The listing builds one solid part. Answer for the finished solid, in the listing's coordinates (mm). Face numbers are marked on the shaded views. A direction names the side the tool comes from. Give positions to 0.01 mm unless a question says otherwise; leave off trailing zeros. Loops run counter-clockwise (first coordinate to the right, second up) from the corner with the lowest first, then second, coordinate; pieces in that order, holes last. Notation, with made-up numbers: (-39.75, -22.75) - (4.25, -22.75) arc R30 ccw to (4.25, 1.25) - close; hole circle Ø4 at (-10, -9.75). An arc over 180 degrees is marked (long way). Answer as CSV lines item,"result". Start each with the question number.
1) A cutting plane is placed at A-A (z = 64.4). Determine the outline of the cut face in (x, y), and give its area (3 significant figures).
2) A cutting plane is placed at C-C (x = -43.5). Determine the outline of the cut face in (y, z), and give its area (3 significant figures).
3) Flat-ended cylindrical pins translate along their axes: pin 1 (2 mm diameter, centred on x = -46, y = 16.5, fed in from +Z); pin 2 (8 mm diameter, centred on y = 12.5, z = 57.4, fed in from -X); pin 3 (3 mm diameter, centred on y = 26.5, z = 49, fed in from +X). Find the tip coordinate at first contact, or state that the pin passes through.
4) A cutting plane is placed at B-B (y = 20). Determine the outline of the cut face in (x, z).
5) Find the intervals of material crossed by line 1 along Z through (x, y) = (-27.9, -1.5); line 2 along Y through (x, z) = (-27.35, 21); line 3 along X through (y, z) = (-2, 53), in increasing order.
6) A cutting plane is placed at D-D (z = 49). Determine the outline of the cut face in (x, y), and give its area (3 significant figures).
7) For a pull along X with two mould halves and no side action, classify the marked faces 4, 5 and 6 as pulls with the +X half, pulls with the -X half, needs draft (parallel to the pull), parting line crosses it, or undercut.
8) For the marked faces 1, 2 and 3, determine the directions among +Z, -Z, +X, -X, +Y, -Y from which every point of the face is accessible in a straight line to the end or side of a thin tool.
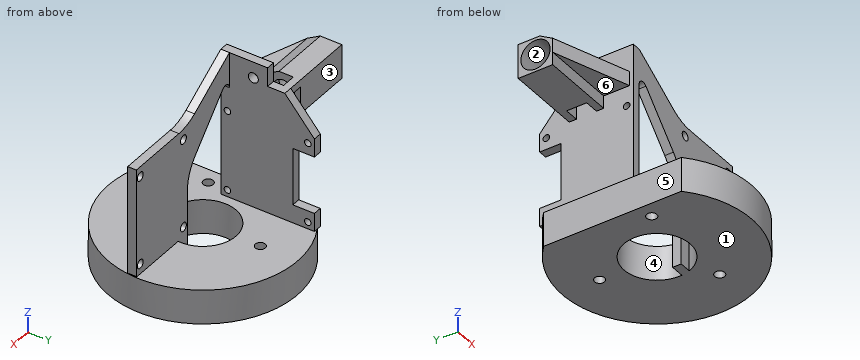
```python
from build123d import *

# Parameters (mm, degrees)
SKETCH_1_R           = 29
EXTRUDE_1_DEPTH      = 5
HOLE_WIZARD_1_D      = 3.5
HOLE_WIZARD_2_D      = 23
EXTRUDE_3_DEPTH      = 65
SKETCH_9_W           = 1
SKETCH_9_H           = 5
CUT_EXTRUDE_1_DEPTH  = 10
SKETCH_10_W          = 3
SKETCH_10_H          = 65
EXTRUDE_5_DEPTH      = 10
HOLE_WIZARD_3_D      = 3.5
EXTRUDE_START        = -65
EXTRUDE_6_DEPTH      = 65
SKETCH_22_W          = 12
SKETCH_22_H          = 6
EXTRUDE_7_DEPTH      = 3
EXTRUDE_8_DEPTH      = 8
HOLE_WIZARD_5_D      = 7
HOLE_WIZARD_5_DEPTH  = 3
SKETCH_27_W          = 5
SKETCH_27_H          = 3.5
CUT_EXTRUDE_3_DEPTH  = 70.598725899
CUT_EXTRUDE_4_REACH  = 94.289
SKETCH_28_W          = 3
SKETCH_28_H          = 3.5
SKETCH_29_R          = 3.5
EXTRUDE_9_DEPTH      = 18
HOLE_WIZARD_6_D      = 10.2
HOLE_WIZARD_6_DEPTH  = 18
SKETCH_32_W          = 26
SKETCH_32_H          = 5
EXTRUDE_10_DEPTH     = 9
CUT_EXTRUDE_5_REACH  = 88.897
SKETCH_36_W          = 32.8
SKETCH_36_H          = 32.6
EXTRUDE_12_DEPTH     = 3
SKETCH_38_R          = 29
CUT_EXTRUDE_7_DEPTH  = 5
SKETCH_39_W          = 17.667068266
SKETCH_39_H          = 15
CUT_EXTRUDE_8_DEPTH  = 13.6
SKETCH_41_R          = 33
EXTRUDE_14_DEPTH     = 12
HOLE_WIZARD_8_D      = 3.5
HOLE_WIZARD_9_D      = 23
HOLE_WIZARD_10_D     = 2.3
SKETCH_53_W          = 20
SKETCH_53_H          = 15
CUT_EXTRUDE_9_DEPTH  = 3
EXTRUDE_16_DEPTH     = 3
SKETCH_56_W          = 3.442096105
SKETCH_56_H          = 51.4
CUT_EXTRUDE_10_DEPTH = 96.777795528
SKETCH_57_W          = 3
SKETCH_57_H          = 1.3
EXTRUDE_17_DEPTH     = 18.6
EXTRUDE_18_DEPTH     = 3
CUT_EXTRUDE_START    = -12
CUT_EXTRUDE_11_DEPTH = 12
SKETCH_63_W          = 26
SKETCH_63_H          = 3
EXTRUDE_21_DEPTH     = 38
HOLE_WIZARD_11_D     = 3
EXTRUDE_22_DEPTH     = 3
CUT_EXTRUDE_START_2  = 4
CUT_EXTRUDE_13_DEPTH = 4
FILLET_1_R           = 15
FILLET_2_R           = 2
EXTRUDE_23_DEPTH     = 12


with BuildPart() as part:
    # 草图1 → 凸台-拉伸1 (new body)
    with BuildSketch(Plane.XY):
        Circle(SKETCH_1_R)
    extrude(amount=EXTRUDE_1_DEPTH)

    # 孔1 (through all)
    with Locations(Plane.XY.offset(5)):
        with Locations((0, 20), (-17.320508076, -10), (17.320508076, -10)):
            Hole(HOLE_WIZARD_1_D / 2)

    # 孔2 (through all)
    with Locations(Plane.XY.offset(5)):
        with Locations((0, 0)):
            Hole(HOLE_WIZARD_2_D / 2)

    # 草图7 → 凸台-拉伸3 (add)
    with BuildSketch(Plane.XY.offset(5)):
        with BuildLine():
            Line((-28.892040426, 2.5), (-28.892040426, -2.5))
            Line((-28.892040426, -2.5), (-11.22497216, -2.5))
            ThreePointArc((-11.22497216, -2.5), (-11.5, 0), (-11.22497216, 2.5))
            Line((-11.22497216, 2.5), (-28.892040426, 2.5))
        make_face()
    extrude(amount=EXTRUDE_3_DEPTH)

    # 草图9 → 切除-拉伸1 (cut)
    with BuildSketch(Plane.XY.offset(5)):
        with Locations((-29.392040426, 0)):
            Rectangle(SKETCH_9_W, SKETCH_9_H)
    extrude(amount=-CUT_EXTRUDE_1_DEPTH, mode=Mode.SUBTRACT)

    # 草图10 → 凸台-拉伸5 (add)
    with BuildSketch(Plane(origin=(0, 2.5, 0), x_dir=(1, 0, 0), z_dir=(0, 1, 0))):
        with Locations((-27.392040426, -37.5)):
            Rectangle(SKETCH_10_W, SKETCH_10_H)
    extrude(amount=EXTRUDE_5_DEPTH)

    # 孔3 (through all)
    with Locations(Plane.ZY.offset(28.892040426)):
        with Locations((10, 7.5), (64.4, 7.5)):
            Hole(HOLE_WIZARD_3_D / 2)

    # 草图20 → 凸台-拉伸6 (add)
    with BuildSketch(Plane.XY.offset(70).offset(EXTRUDE_START)):
        with BuildLine():
            Line((-11.22497216, 2.5), (-11.22497216, -2.5))
            ThreePointArc((-11.22497216, -2.5), (-11.5, 0), (-11.22497216, 2.5))
        make_face()
    extrude(amount=EXTRUDE_6_DEPTH)

    # 草图22 → 凸台-拉伸7 (add)
    with BuildSketch(Plane.ZY.offset(28.892040426)):
        with Locations((57.4, 15.5)):
            Rectangle(SKETCH_22_W, SKETCH_22_H)
    extrude(amount=-EXTRUDE_7_DEPTH)

    # 草图23 → 凸台-拉伸8 (add)
    with BuildSketch(Plane.ZY.offset(28.892040426)):
        Polygon((51.4, 6.5), (60.801923789, 6.5), (63.4, 11), (63.4, 12.5), (63.4, 18.5), (51.4, 18.5), (51.4, 12.5), align=None)
    extrude(amount=EXTRUDE_8_DEPTH)

    # 孔5
    with Locations(Plane.ZY.offset(36.892040426)):
        with Locations((57.4, 12.5)):
            Hole(HOLE_WIZARD_5_D / 2, depth=HOLE_WIZARD_5_DEPTH)

    # 草图27 → 切除-拉伸3 (cut, through all)
    with BuildSketch(Plane(origin=(0, 0, 51.4), x_dir=(-1, 0, 0), z_dir=(0, 0, -1))):
        with Locations((31.392040426, 14.25)):
            Rectangle(SKETCH_27_W, SKETCH_27_H)
        with Locations((31.392040426, 10.75)):
            Rectangle(SKETCH_27_W, SKETCH_27_H)
    extrude(amount=-CUT_EXTRUDE_3_DEPTH, mode=Mode.SUBTRACT)

    # 草图28 → 切除-拉伸4 (cut, up to next)
    with BuildSketch(Plane(origin=(0, 18.5, 0), x_dir=(1, 0, 0), z_dir=(0, 1, 0)), mode=Mode.PRIVATE) as cut_extrude_4_sk1:
        with Locations((-32.392040426, -59.15)):
            Rectangle(SKETCH_28_W, SKETCH_28_H)
    cut_extrude_4_tool1 = extrude(cut_extrude_4_sk1.sketch, amount=-CUT_EXTRUDE_4_REACH, mode=Mode.PRIVATE) & part.part
    # 草图28 → 切除-拉伸4 (cut, up to next)
    with BuildSketch(Plane(origin=(0, 18.5, 0), x_dir=(1, 0, 0), z_dir=(0, 1, 0)), mode=Mode.PRIVATE) as cut_extrude_4_sk2:
        with Locations((-32.392040426, -55.65)):
            Rectangle(SKETCH_28_W, SKETCH_28_H)
    cut_extrude_4_tool2 = extrude(cut_extrude_4_sk2.sketch, amount=-CUT_EXTRUDE_4_REACH, mode=Mode.PRIVATE) & part.part
    add(cut_extrude_4_tool1.solids().sort_by_distance((-32.39204, 18.5, 59.15))[0], mode=Mode.SUBTRACT)
    add(cut_extrude_4_tool2.solids().sort_by_distance((-32.39204, 18.5, 55.65))[0], mode=Mode.SUBTRACT)

    # 草图29 → 凸台-拉伸9 (add)
    # profile 1 of 2: a face of its own
    with BuildSketch(Plane.ZY.offset(36.892040426)):
        Polygon((60.801923789, 6.5), (63.4, 11), (63.4, 18.5), (51.4, 18.5), (51.4, 6.5), align=None)
        with Locations((57.4, 12.5)):
            Circle(SKETCH_29_R, mode=Mode.SUBTRACT)
    # profile 2 of 2: a face of its own
    with BuildSketch(Plane.ZY.offset(36.892040426)):
        with Locations((57.4, 12.5)):
            Circle(SKETCH_29_R)
    extrude(amount=EXTRUDE_9_DEPTH)

    # 孔6
    with Locations(Plane.ZY.offset(54.892040426)):
        with Locations((57.4, 12.5)):
            Hole(HOLE_WIZARD_6_D / 2, depth=HOLE_WIZARD_6_DEPTH)

    # 草图32 → 凸台-拉伸10 (add)
    with BuildSketch(Plane.XZ.offset(-6.5)):
        with Locations((-41.892040426, 58.301923789)):
            Rectangle(SKETCH_32_W, SKETCH_32_H)
    extrude(amount=EXTRUDE_10_DEPTH)

    # 草图33 → 切除-拉伸5 (cut, up to next)
    with BuildSketch(Plane.XY.offset(60.801923789), mode=Mode.PRIVATE) as cut_extrude_5_sk1:
        Polygon((-54.892040426, 6.5), (-28.892040426, -2.5), (-54.892040426, -2.5), align=None)
    cut_extrude_5_tool1 = extrude(cut_extrude_5_sk1.sketch, amount=-CUT_EXTRUDE_5_REACH, mode=Mode.PRIVATE) & part.part
    add(cut_extrude_5_tool1.solids().sort_by_distance((-46.225374, 0.5, 60.801924))[0], mode=Mode.SUBTRACT)

    # 草图36 → 凸台-拉伸12 (add)
    with BuildSketch(Plane.ZY.offset(28.892040426)):
        with Locations((35, 12.5)):
            Rectangle(SKETCH_36_W, SKETCH_36_H)
    extrude(amount=-EXTRUDE_12_DEPTH)

    # 草图38 → 切除-拉伸7 (cut)
    with BuildSketch(Plane(origin=(0, 0, 0), x_dir=(-1, 0, 0), z_dir=(0, 0, -1))):
        Circle(SKETCH_38_R)
    extrude(amount=-CUT_EXTRUDE_7_DEPTH, mode=Mode.SUBTRACT)

    # 草图39 → 切除-拉伸8 (cut)
    with BuildSketch(Plane(origin=(0, 0, 5), x_dir=(-1, 0, 0), z_dir=(0, 0, -1))):
        with Locations((20.058506293, 5)):
            Rectangle(SKETCH_39_W, SKETCH_39_H)
    extrude(amount=-CUT_EXTRUDE_8_DEPTH, mode=Mode.SUBTRACT)

    # 草图41 → 凸台-拉伸14 (add)
    with BuildSketch(Plane(origin=(0, 0, 18.6), x_dir=(-1, 0, 0), z_dir=(0, 0, -1))):
        with Locations(Location((11.22497216, 0, 0), (0, 0, 57.631283974))):
            Circle(SKETCH_41_R)
    extrude(amount=EXTRUDE_14_DEPTH)

    # 孔8 (through all)
    with Locations(Plane(origin=(0, 0, 6.6), x_dir=(-1, 0, 0), z_dir=(0, 0, -1))):
        with Locations((11.22497216, 20), (-6.095535915, -10), (28.545480236, -10)):
            Hole(HOLE_WIZARD_8_D / 2)

    # 孔9 (through all)
    with Locations(Plane(origin=(0, 0, 6.6), x_dir=(-1, 0, 0), z_dir=(0, 0, -1))):
        with Locations((11.22497216, 0)):
            Hole(HOLE_WIZARD_9_D / 2)

    # 孔10 (through all)
    with Locations(Plane.ZY.offset(28.892040426)):
        with Locations((21, 26.5), (49, 26.5), (49, -1.5), (21, -1.5)):
            Hole(HOLE_WIZARD_10_D / 2)

    # 草图53 → 切除-拉伸9 (cut)
    with BuildSketch(Plane.ZY.offset(28.892040426)):
        with Locations((35, 28.8)):
            Rectangle(SKETCH_53_W, SKETCH_53_H)
    extrude(amount=-CUT_EXTRUDE_9_DEPTH, mode=Mode.SUBTRACT)

    # 草图55 → 凸台-拉伸16 (add)
    with BuildSketch(Plane(origin=(-25.892040426, 0, 0), x_dir=(0, 0, -1), z_dir=(1, 0, 0))):
        Polygon((-51.4, 28.8), (-63.4, 18.5), (-51.4, 18.5), align=None)
    extrude(amount=-EXTRUDE_16_DEPTH)

    # 草图56 → 切除-拉伸10 (cut, through all)
    with BuildSketch(Plane(origin=(0, 2.5, 0), x_dir=(1, 0, 0), z_dir=(0, 1, 0))):
        with Locations((-24.170992373, -44.3)):
            Rectangle(SKETCH_56_W, SKETCH_56_H)
    extrude(amount=-CUT_EXTRUDE_10_DEPTH, mode=Mode.SUBTRACT)

    # 草图57 → 凸台-拉伸17 (add)
    with BuildSketch(Plane.XY.offset(51.4)):
        with Locations((-27.392040426, -3.15)):
            Rectangle(SKETCH_57_W, SKETCH_57_H)
    extrude(amount=EXTRUDE_17_DEPTH)

    # 草图58 → 凸台-拉伸18 (add)
    with BuildSketch(Plane.XZ.offset(3.8)):
        Polygon((-25.892040426, 70), (21.77502784, 18.6), (14.955892727, 18.6), (-25.892040426, 62.646840732), align=None)
    extrude(amount=-EXTRUDE_18_DEPTH)

    # 草图62 → 切除-拉伸11 (cut)
    with BuildSketch(Plane(origin=(0, 0, 6.6), x_dir=(-1, 0, 0), z_dir=(0, 0, -1)).offset(CUT_EXTRUDE_START)):
        Polygon((33.892040426, 193.306123394), (33.892040426, 23.983411272), (33.892040426, -23.983411272), (33.892040426, -193.306123394), (372.537464671, -193.306123394), (372.537464671, 193.306123394), align=None)
    extrude(amount=CUT_EXTRUDE_11_DEPTH, mode=Mode.SUBTRACT)

    # 草图63 → 凸台-拉伸21 (add)
    with BuildSketch(Plane.XY.offset(18.6)):
        with Locations((8.555509837, -2.3)):
            Rectangle(SKETCH_63_W, SKETCH_63_H)
    extrude(amount=EXTRUDE_21_DEPTH)

    # 孔11 (through all)
    with Locations(Plane(origin=(0, -0.8, 0), x_dir=(1, 0, 0), z_dir=(0, 1, 0))):
        with Locations((-2.444490163, -22.1), (19.555509837, -22.1), (-2.444490163, -53.1), (19.555509837, -53.1)):
            Hole(HOLE_WIZARD_11_D / 2)

    # 草图67 → 凸台-拉伸22 (add)
    with BuildSketch(Plane(origin=(0, -0.8, 0), x_dir=(1, 0, 0), z_dir=(0, 1, 0))):
        Polygon((-25.892040426, -70), (-4.444490163, -56.6), (-4.444490163, -46.872836454), align=None)
    extrude(amount=-EXTRUDE_22_DEPTH)

    # 草图68 → 切除-拉伸13 (cut)
    with BuildSketch(Plane.XY.offset(18.6).offset(CUT_EXTRUDE_START_2)):
        with BuildLine():
            ThreePointArc((21.555509837, -3.8), (21.498484695, -4.263258313), (21.434913054, -4.725663739))
            Line((21.434913054, -4.725663739), (29.536238519, -6.781789189))
            ThreePointArc((29.536238519, -6.781789189), (29.956240846, -3.402448529), (30.096559281, 0))
            ThreePointArc((30.096559281, 0), (30.084776458, 0.986726755), (30.049434711, 1.972890781))
            Line((30.049434711, 1.972890781), (21.716000836, 1.972890781))
            ThreePointArc((21.716000836, 1.972890781), (21.760267788, 0.9868868), (21.77502784, 0))
            ThreePointArc((21.77502784, 0), (21.772603152, -0.400029392), (21.765329445, -0.8))
            ThreePointArc((21.765329445, -0.8), (21.694611585, -2.30239138), (21.555509837, -3.8))
        make_face()
    extrude(amount=-CUT_EXTRUDE_13_DEPTH, mode=Mode.SUBTRACT)

    # 圆角1
    fillet_1_edges = [part.edges().sort_by_distance(p)[0] for p in [
        (-4.444490163, -2.3, 56.6),
        (-4.444490163, -2.3, 39.519677186),
    ]]
    fillet(fillet_1_edges, radius=FILLET_1_R)

    # 圆角2
    fillet_2_edges = [part.edges().sort_by_distance(p)[0] for p in [
        (-25.892040426, -2.3, 62.646840732),
    ]]
    fillet(fillet_2_edges, radius=FILLET_2_R)

    # 草图69 → 凸台-拉伸23 (add)
    with BuildSketch(Plane(origin=(0, 0, 18.6), x_dir=(-1, 0, 0), z_dir=(0, 0, -1))):
        with BuildLine():
            Line((4.444490163, -3.8), (4.444490163, -0.8))
            Line((4.444490163, -0.8), (-0.247168006, -0.8))
            ThreePointArc((-0.247168006, -0.8), (-0.038441417, -2.320671148), (0.370940651, -3.8))
            Line((0.370940651, -3.8), (4.444490163, -3.8))
        make_face()
    extrude(amount=EXTRUDE_23_DEPTH)


solid = part.part
```
Ans:
1,outline,"(-28.89, -3.8) - (-16.93, -3.8) - (-16.93, -0.8) - (-25.89, -0.8) - (-25.89, 5.75) - (-28.89, 5.75) - close; (-28.89, 9.25) - (-25.89, 9.25) - (-25.89, 12.5) - (-28.89, 12.5) - close"
1,area,"65.3 mm2"
2,outline,"(2.56, 55.8) - (6.5, 55.8) - (6.5, 51.4) - (18.5, 51.4) - (18.5, 63.4) - (11, 63.4) - (6.5, 60.8) - (2.56, 60.8) - close; hole circle Ø10.2 at (12.5, 57.4)"
2,area,"76.2 mm2"
3,pin 1,"z = 63.4"
3,pin 2,"x = -36.89"
3,pin 3,"x = -25.89"
4,outline,"(-33.89, 6.6) - (-12.97, 6.6) - (-12.97, 18.6) - (-25.89, 18.6) - (-25.89, 61.65) - (-28.89, 61.65) - (-28.89, 18.6) - (-33.89, 18.6) - close; (-9.47, 6.6) - (15.02, 6.6) - (15.02, 18.6) - (-9.47, 18.6) - close"
5,line 1,"6.6 to 19.85, 22.15 to 47.85, 50.15 to 70"
5,line 2,"-3.8 to -2.65, -0.35 to 25.35, 27.65 to 28.8"
5,line 3,"-28.89 to -25.89, -16.95 to -3.94, -0.95 to 18.06, 21.05 to 21.56"
6,outline,"(-28.89, -3.8) - (-25.89, -3.8) - (-25.89, -2.65) - (-28.89, -2.65) - close; (-28.89, -0.35) - (-25.89, -0.35) - (-25.89, 25.35) - (-28.89, 25.35) - close; (-28.89, 27.65) - (-25.89, 27.65) - (-25.89, 28.8) - (-28.89, 28.8) - close; (-13.24, -3.8) - (21.56, -3.8) - (21.56, -0.8) - (-13.24, -0.8) - close"
6,area,"188 mm2"
7,face 4,"undercut"
7,face 5,"pulls with the -X half"
7,face 6,"needs draft"
8,face 1,"-Z, +X, -X, +Y, -Y"
8,face 2,"-X"
8,face 3,"+Z, -X, +Y"
